Solid Edge part; units mm, degrees
sketch "Sketch1" plane through (0, 0, 0) normal (1, 0, 0) x (0, 1, 0)
  line L0 (27.5, -27) -> (27.5, 23)
  line L1 (27.5, 23) -> (-31.5, 23)
  line L2 (-31.5, 23) -> (-31.5, -27)
  line L3 (-31.5, -27) -> (27.5, -27)
extrude "Protrusion1" add sketch "Sketch1" along normal blind 2
sketch "Sketch2" plane through (0, 0, 0) normal (1, 0, 0) x (0, 1, 0)
  line L0 (-31.5, 21) -> (-7, 21)
  line L1 (-7, 21) -> (-7, 23)
  line L2 (-7, 23) -> (-31.5, 23)
  line L3 (-31.5, 23) -> (-31.5, 21)
extrude "ExtrudedCutout_1" cut sketch "Sketch2" along normal blind 2
sketch "Sketch3" plane through (0, 0, 0) normal (1, 0, 0) x (0, 1, 0)
  line L0 (3, 21) -> (27.5, 21)
  line L1 (27.5, 21) -> (27.5, 23)
  line L2 (27.5, 23) -> (3, 23)
  line L3 (3, 23) -> (3, 21)
extrude "ExtrudedCutout_2" cut sketch "Sketch3" along normal blind 2
sketch "Sketch4" plane through (0, 0, 0) normal (1, 0, 0) x (0, 1, 0)
  line L0 (23.5, 3) -> (23.5, -7)
  line L1 (23.5, -7) -> (25.5, -7)
  line L2 (25.5, -7) -> (25.5, 3)
  line L3 (25.5, 3) -> (23.5, 3)
extrude "ExtrudedCutout_3" cut sketch "Sketch4" along normal blind 2
sketch "Sketch5" plane through (0, 0, 0) normal (1, 0, 0) x (0, 1, 0)
  line L0 (27.5, -25) -> (3, -25)
  line L1 (3, -25) -> (3, -27)
  line L2 (3, -27) -> (27.5, -27)
  line L3 (27.5, -27) -> (27.5, -25)
extrude "ExtrudedCutout_4" cut sketch "Sketch5" along normal blind 4
sketch "Sketch6" plane through (0, 0, 0) normal (1, 0, 0) x (0, 1, 0)
  line L0 (-7, -25) -> (-31.5, -25)
  line L1 (-31.5, -25) -> (-31.5, -27)
  line L2 (-31.5, -27) -> (-7, -27)
  line L3 (-7, -27) -> (-7, -25)
extrude "ExtrudedCutout_5" cut sketch "Sketch6" along normal blind 2
sketch "Sketch7" plane through (0, 0, 0) normal (1, 0, 0) x (0, 1, 0)
  line L0 (-29.5, -7) -> (-27.5, -7)
  line L1 (-27.5, -7) -> (-27.5, 3)
  line L2 (-27.5, 3) -> (-29.5, 3)
  line L3 (-29.5, 3) -> (-29.5, -7)
extrude "ExtrudedCutout_6" cut sketch "Sketch7" along normal blind 4
sketch "Sketch8" plane through (0, 0, 0) normal (1, 0, 0) x (0, 1, 0)
  circle A0 centre (-11.5, 10) radius 1.6
  circle A1 centre (7.5, -14) radius 1.6
extrude "ExtrudedCutout_7" cut sketch "Sketch8" along normal blind 2
fillet "Round_1" radius 1 4 edges at (1, 27.5, -25) (1, 27.5, 21) (1, -31.5, 21) (1, -31.5, -25)
properties material "Acrylic, high impact grade"
Could you check a few things on this model? Use its own coordinates, in mm. A direction names the side the tool comes from. Coordinates: 2 decimals unless noted, no trailing zeros. Write each loop counter-clockwise with the first axis right and the second up, starting at its lowest first coordinate (ties: lowest second). Pieces come first, ordered by that corner, then holes. Notation, with made-up numbers: (23, -8) - (55, -8) arc R9 cw to (55, -1) - close; hole circle Ø1 at (-6, 46.25). An arc over 180 degrees is marked (long way). Use a Markdown table: item, result.
Q1. I'm going to push flat-ended pins straight in: pin 1 Ø1 at (x, y) = (1.5, 24.5) entering from +Z; pin 2 Ø2 at (y, z) = (-10.5, 17.5) entering from -X; pin 3 Ø1 at (x, y) = (1, 24.5) entering from -Z; pin 4 Ø1 at (x, z) = (1.5, 22.5) entering from -Y. Where does each tip first touch, or does it pass through?
Geometry check:
| item | result |
|---|---|
| pin 1 | stops at z = 21 |
| pin 2 | stops at x = 0 |
| pin 3 | stops at z = -25 |
| pin 4 | stops at y = -7 |
Q2. Thinking about a two-plate mould opening in Z: for faces 5 (the flat face through (1, 24, -7)), 6 (the flat face through (1, -29.5, -2)), 7 (the flat face through (1, 27.5, -2)), 8 (the flat face through (1, 15, -25)), which applies, +Z half, -Z half, draft (parallel to the pull), parting line (faces both ways), or undercut?
Geometry check:
| item | result |
|---|---|
| face 5 | undercut |
| face 6 | undercut |
| face 7 | draft |
| face 8 | -Z half |
Q3. Imagine slicing it at B-B (x = 1.7). List the corners of the cut face in (y, z) for me, and give its area (3 significant figures).
Geometry check:
| item | result |
|---|---|
| outline | (-31.5, -24) arc R1 ccw to (-30.5, -25) - (-7, -25) - (-7, -27) - (3, -27) - (3, -25) - (26.5, -25) arc R1 ccw to (27.5, -24) - (27.5, 20) arc R1 ccw to (26.5, 21) - (3, 21) - (3, 23) - (-7, 23) - (-7, 21) - (-30.5, 21) arc R1 ccw to (-31.5, 20) - close; hole (-29.5, -7) - (-27.5, -7) - (-27.5, 3) - (-29.5, 3) - close; hole circle Ø3.2 at (-11.5, 10); hole circle Ø3.2 at (7.5, -14); hole (23.5, -7) - (25.5, -7) - (25.5, 3) - (23.5, 3) - close |
| area | 2,700 mm2 |
Q4. Imagine slicing it at D-D (z = -2.5). List the corners of the cut face in (x, y) for me.
Geometry check:
| item | result |
|---|---|
| outline | (0, -31.5) - (2, -31.5) - (2, -29.5) - (0, -29.5) - close; (0, -27.5) - (2, -27.5) - (2, 23.5) - (0, 23.5) - close; (0, 25.5) - (2, 25.5) - (2, 27.5) - (0, 27.5) - close |
Q5. Please list where these lines run through material, in increasing order: L1, parallel to Y at x = 1.05, z = -2.5; L2, parallel to Z at x = 1.2, y = 7.5; L3, parallel to Z at x = 1.5, y = -11.5.
Geometry check:
| item | result |
|---|---|
| L1 | y = -31.5 to -29.5, -27.5 to 23.5, 25.5 to 27.5 |
| L2 | z = -25 to -15.6, -12.4 to 21 |
| L3 | z = -25 to 8.4, 11.6 to 21 |
Q6. Imagine slicing it at C-C (y = 7.5). List the corners of the cut face in (x, z) for me, and give its area (3 significant figures).
Geometry check:
| item | result |
|---|---|
| outline | (0, -25) - (2, -25) - (2, -15.6) - (0, -15.6) - close; (0, -12.4) - (2, -12.4) - (2, 21) - (0, 21) - close |
| area | 85.6 mm2 |
Q7. Which directions (+Z, -Z, +X, -X, +Y, -Y) give clear straight access to the entire face, cutting with the end or side of a thin tool? Please do faces 1 (the flat face through (1, 15, 21)), 2 (the flat face through (1, 25.5, -2)), 3 (the flat face through (1, -7, 22)), 4 (the flat face through (1, -7, -26)).
Geometry check:
| item | result |
|---|---|
| face 1 | +Z, +X, -X, +Y |
| face 2 | +X, -X |
| face 3 | +Z, +X, -X, -Y |
| face 4 | -Z, +X, -X, -Y |
Q8. Imagine slicing it at A-A (z = 10). List the corners of the cut face in (x, y) for me.
Geometry check:
| item | result |
|---|---|
| outline | (0, -31.5) - (2, -31.5) - (2, -13.1) - (0, -13.1) - close; (0, -9.9) - (2, -9.9) - (2, 27.5) - (0, 27.5) - close |
